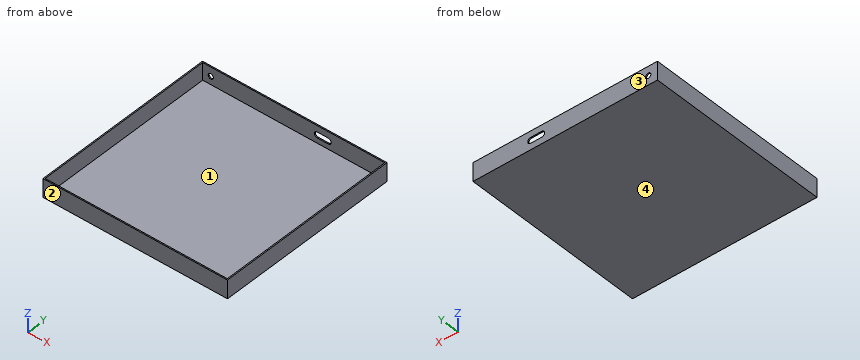
from build123d import *

# Parameters (mm, degrees)
SKETCH1_W           = 508
SKETCH1_H           = 508
BOSS_EXTRUDE1_DEPTH = 50.8
SHELL1_T            = -3.175
SKETCH2_R           = 7.14375
CUT_EXTRUDE1_DEPTH  = 417.576


with BuildPart() as part:
    # Sketch1 → Boss-Extrude1 (new body)
    with BuildSketch(Plane.XY):
        with Locations((254, 254)):
            Rectangle(SKETCH1_W, SKETCH1_H)
    extrude(amount=BOSS_EXTRUDE1_DEPTH)

    # Shell1
    shell1_openings = [part.faces().sort_by_distance(p)[0] for p in [
        (254, 254, 50.8),
    ]]
    offset(amount=SHELL1_T, openings=shell1_openings, kind=Kind.INTERSECTION)

    # Sketch2 → Cut-Extrude1 (cut)
    with BuildSketch(Plane(origin=(0, 508, 0), x_dir=(1, 0, 0), z_dir=(0, 1, 0))):
        with Locations(Location((25.4, -25.4, 0), (0, 0, 270))):
            Circle(SKETCH2_R)
        with BuildLine():
            Line((349.25, -33.3375), (318.77, -33.3375))
            ThreePointArc((318.77, -33.3375), (310.8325, -25.4), (318.77, -17.4625))
            Line((318.77, -17.4625), (349.25, -17.4625))
            ThreePointArc((349.25, -17.4625), (357.1875, -25.4), (349.25, -33.3375))
        make_face()
    extrude(amount=-CUT_EXTRUDE1_DEPTH, mode=Mode.SUBTRACT)


solid = part.part
Design review of the part built by this model. Coordinates are the model's own, in mm. Face numbers are marked on the shaded views. Coordinates: 2 decimals unless noted, no trailing zeros. Order: outer loops, then holes, each group sorted by start corner. A loop starts at its lowest first (then second) coordinate and runs counter-clockwise, first axis right, second up.
Item 1: Take a section at B-B, the plane y = 476.5. Write out the cut boundary in (x, z) (3 decimals).
Item 2: For line 1 (X direction, y = 506, z = 25); line 2 (Y direction, x = 186, z = 16.5) (3 decimals); line 3 (Z direction, x = 25, y = 507), list the stretches that pass through material, from the lowest coordinate up.
Item 3: Take a section at A-A, the plane z = 25.4. Write out the cut boundary in (x, y) (1 decimal).
Item 4: For pin 1 Ø3 at (x, y) = (166.5, 110.5) entering from -Z; pin 2 Ø3 at (x, z) = (334.5, 21) entering from +Y (3 decimals), all flat-tipped, find the tip position at first contact; note any pin that passes through.
Item 5: The part is to be moulded in two halves that separate along Y. For the marked faces 1, 2, 3 and 4, say which applies: pulls with the +Y half, pulls with the -Y half, needs draft (parallel to the pull), parting line crosses it, or undercut.
The answers:
1. outline: (0, 0) - (508, 0) - (508, 50.8) - (504.825, 50.8) - (504.825, 3.175) - (3.175, 3.175) - (3.175, 50.8) - (0, 50.8) - close
2. line 1: x = 0 to 18.27, 32.53 to 310.84, 357.18 to 508
2. line 2: y = 0 to 3.175, 504.825 to 508
2. line 3: z = 0 to 18.27, 32.53 to 50.8
3. outline: (0, 0) - (508, 0) - (508, 508) - (357.2, 508) - (357.2, 504.8) - (504.8, 504.8) - (504.8, 3.2) - (3.2, 3.2) - (3.2, 504.8) - (18.3, 504.8) - (18.3, 508) - (0, 508) - close; (32.5, 504.8) - (310.8, 504.8) - (310.8, 508) - (32.5, 508) - close
4. pin 1: stops at z = 0
4. pin 2: stops at y = 3.175
5. face 1: undercut
5. face 2: pulls with the -Y half
5. face 3: pulls with the +Y half
5. face 4: needs draft
